```python
from build123d import *

# Parameters (mm, degrees)
SKETCH1_W                 = 42
SKETCH1_H                 = 42
BOSS_EXTRUDE1_DEPTH       = 33.02
M3X0_5_TAPPED_HOLE1_D     = 2.5
M3X0_5_TAPPED_HOLE1_DEPTH = 7.5
M3X0_5_TAPPED_HOLE1_TIP   = 0.751075774
FILLET1_R                 = 3.175


with BuildPart() as part:
    # Sketch1 → Boss-Extrude1 (new body)
    with BuildSketch(Plane.XY.offset(33.02)):
        Rectangle(SKETCH1_W, SKETCH1_H)
    extrude(amount=-BOSS_EXTRUDE1_DEPTH)

    # Sketch6 → Revolve5 (revolve)
    with BuildSketch(Plane(origin=(0, 0, 0), x_dir=(1, 0, 0), z_dir=(0, 1, 0))):
        Polygon((10.9982, -33.02), (0, -33.02), (0, -45.72), (2.5, -45.72), (2.5, -35.02), (10.9982, -35.02), align=None)
    revolve(axis=Axis((0, 0, 33.02), (0, 0, 1)))

    # M3x0.5 Tapped Hole1
    with Locations(Plane.XY.offset(33.02)):
        with Locations((-15.5, 15.5), (-15.5, -15.5), (15.5, -15.5), (15.5, 15.5)):
            Hole(M3X0_5_TAPPED_HOLE1_D / 2, depth=M3X0_5_TAPPED_HOLE1_DEPTH)
            with Locations((0, 0, -(M3X0_5_TAPPED_HOLE1_DEPTH + M3X0_5_TAPPED_HOLE1_TIP / 2))):  # 118° drill point
                Cone(0, M3X0_5_TAPPED_HOLE1_D / 2, M3X0_5_TAPPED_HOLE1_TIP, mode=Mode.SUBTRACT)

    # Fillet1
    fillet1_edges = [part.edges().sort_by_distance(p)[0] for p in [
        (-21, -21, 16.51),
        (-21, 21, 16.51),
        (21, 21, 16.51),
        (21, -21, 16.51),
    ]]
    fillet(fillet1_edges, radius=FILLET1_R)


solid = part.part
```
CAD build for the part. Positions are in the model's coordinates, mm. A direction names the side the tool comes from. Round coordinates to 2 decimals unless told otherwise and drop trailing zeros. Order: outer loops, then holes, each group sorted by start corner. A loop starts at its lowest first (then second) coordinate and runs counter-clockwise, first axis right, second up.
Item 1: Mould opens along X. For faces 3 (the face through (20.05, -20.09, 16.28)), 4 (the face through (-14.579, 16.345, 29.218)), 5 (the face through (0, 3, 35.02)), 6 (the face through (-0.54, -2.44, 40.3)) say: pulls with the +X half, pulls with the -X half, needs draft (parallel to the pull), parting line crosses it, or undercut.
Item 2: Probe line 1 along Y through (x, z) = (-15.5, 30); line 2 along Y through (x, z) = (-15, 28). List the from-to ranges inside material, lowest first.
Item 3: Saw through at B-B on x = 0. Write the cut outline in (y, z).
Item 4: Tool access for faces 1 (the face through (0, 21, 17)), 2 (the face through (-15.34, -14.26, 29.22)): list every direction of +Z, -Z, +X, -X, +Y, -Y with a clear straight run to the whole face (end or side of a thin tool).
Item 5: Pin check, flat tip, straight feed: pin 1 (2 mm diameter, centred on x = -15.5, y = 15.5, fed in from +Z). Stop position of the tip, or through.
Item 6: Saw through at A-A on z = 29. Write the cut outline in (x, y) (3 decimals), then the cut area to 3 significant figures.
Item 7: Saw through at D-D on x = 8. Write the cut outline in (y, z).
Reported:
1. face 3: pulls with the +X half
1. face 4: undercut
1. face 5: needs draft
1. face 6: parting line crosses it
2. line 1: y = -21 to -16.75, -14.25 to 14.25, 16.75 to 21
2. line 2: y = -21 to -16.65, -14.35 to 14.35, 16.65 to 21
3. outline: (-21, 0) - (21, 0) - (21, 33.02) - (11, 33.02) - (11, 35.02) - (2.5, 35.02) - (2.5, 45.72) - (-2.5, 45.72) - (-2.5, 35.02) - (-11, 35.02) - (-11, 33.02) - (-21, 33.02) - close
4. face 1: +Z, -Z, +X, -X, +Y
4. face 2: +Z
5. pin 1: stops at z = 25.37
6. outline: (-21, -17.825) arc R3.175 ccw to (-17.825, -21) - (17.825, -21) arc R3.175 ccw to (21, -17.825) - (21, 17.825) arc R3.175 ccw to (17.825, 21) - (-17.825, 21) arc R3.175 ccw to (-21, 17.825) - close; hole circle Ø2.5 at (-15.5, -15.5); hole circle Ø2.5 at (-15.5, 15.5); hole circle Ø2.5 at (15.5, -15.5); hole circle Ø2.5 at (15.5, 15.5)
6. area: 1,740 mm2
7. outline: (-21, 0) - (21, 0) - (21, 33.02) - (7.55, 33.02) - (7.55, 35.02) - (-7.55, 35.02) - (-7.55, 33.02) - (-21, 33.02) - close
